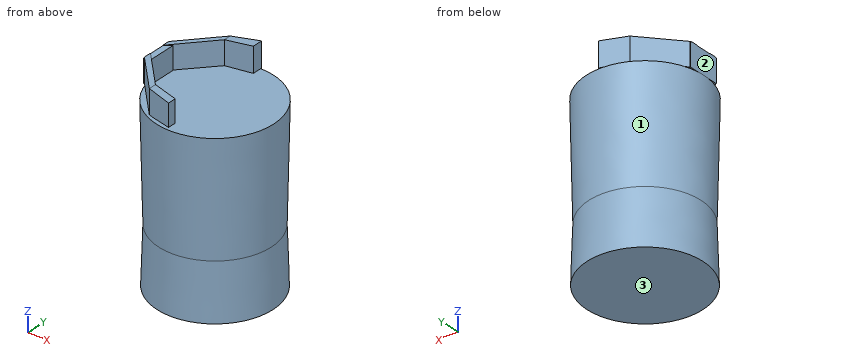
```python
from build123d import *

# Parameters (mm, degrees)
F10_R      = 51.6766678949
F9_R       = 49.5177054899
F14_R      = 51.0900787087
F11_FACE_R = 49.5177054899
F17_W      = 28.0700735748
F17_H      = 20.5879807472
F20_W      = 25.325415656
F20_H      = 19.9093073606
F23_W      = 6.3016116619
F23_H      = 20.8089984953
F22_W      = 6.4192367718
F22_H      = 20.5292478204
F22_W_2    = 6.6290111281
F22_H_2    = 20.7466594875
F23_W_2    = 6.6997222602
F23_H_2    = 21.3462822139
F26_W      = 7.3063448071
F26_H      = 19.5261649787
F28_W      = 9.0555027127
F28_H      = 21.7844322324


with BuildPart() as f11:
    # F10 (on face) → F11 section 0
    with BuildSketch(Plane.XY.offset(50.2420156263)):
        Circle(F10_R)
    # F9 (on face) → F11 section 1
    with BuildSketch(Plane.XY.offset(-49.2490320466)):
        Circle(F9_R)
    loft()

    # F14 (on offset) → F15 section 0
    with BuildSketch(Plane.XY.offset(-98.71355223)):
        Circle(F14_R)
    # F11_face (on face) → F15 section 1
    with BuildSketch(Plane(origin=(0, 0, -49.2490320466), x_dir=(1, 0, 0), z_dir=(0, 0, -1))):
        Circle(F11_FACE_R)
    loft()

    # F17 (on offset) → F21 section 0
    with BuildSketch(Plane.YZ.offset(-51.4408089221)):
        with Locations((-0.1785028726, 60.4957193136)):
            Rectangle(F17_W, F17_H)
    # F20 (on offset) → F21 section 1
    with BuildSketch(Plane.YZ.offset(-46.7405449599)):
        with Locations((-0.1616971567, 60.256190598)):
            Rectangle(F20_W, F20_H)
    loft()

    # F23 (on offset) → F24 section 0
    with BuildSketch(Plane.YZ.offset(-22.4701166153)):
        with Locations((41.3124375045, 61.3829698414)):
            Rectangle(F23_W, F23_H)
    # F22 (on offset) → F24 section 1
    with BuildSketch(Plane.YZ.offset(-51.4408089221)):
        with Locations((9.9052698351, 60.8711652458)):
            Rectangle(F22_W, F22_H)
    loft()

    # F22 (on offset) → F25 section 0
    with BuildSketch(Plane.YZ.offset(-51.4408089221)):
        with Locations((-10.0758362096, 60.7760790735)):
            Rectangle(F22_W_2, F22_H_2)
    # F23 (on offset) → F25 section 1
    with BuildSketch(Plane.YZ.offset(-22.4701166153)):
        with Locations((-40.5898671597, 60.6302414089)):
            Rectangle(F23_W_2, F23_H_2)
    loft()

    # F23 (on offset) → F27 section 0
    with BuildSketch(Plane.YZ.offset(-22.4701166153)):
        with Locations((-40.5898671597, 60.6302414089)):
            Rectangle(F23_W_2, F23_H_2)
    # F26 (on Right) → F27 section 1
    with BuildSketch(Plane.YZ):
        with Locations((-47.1889227629, 61.6251770407)):
            Rectangle(F26_W, F26_H)
    loft()

    # F28 (on Right) → F29 section 0
    with BuildSketch(Plane.YZ):
        with Locations((46.41026631, 62.4425597489)):
            Rectangle(F28_W, F28_H)
    # F23 (on offset) → F29 section 1
    with BuildSketch(Plane.YZ.offset(-22.4701166153)):
        with Locations((41.3124375045, 61.3829698414)):
            Rectangle(F23_W, F23_H)
    loft()


solid = f11.part
```
Geometry check sheet. Reference: the model listing, model coordinates, mm. Face numbers are marked on the shaded views. Round coordinates to 2 decimals unless told otherwise and drop trailing zeros. Order: outer loops, then holes, each group sorted by start corner. A loop starts at its lowest first (then second) coordinate and runs counter-clockwise, first axis right, second up. Notation, with made-up numbers: (-13.75, -17) -> (33.25, -17) arc R10 cw to (33.25, -7) -> close; hole circle Ø2 at (-13, 81). An arc over 180 degrees is marked (long way). Return JSON: item names as keys, results as strings. Group by question number.
Q1. Section check B-B, the plane z = 15. Record the boundary of the cut face in (x, y), plus the area to 3 significant figures.
Q2. Gauge pin test, flat ends, axial feed: pin 1 (1.5 mm diameter, centred on x = -22.5, z = 12, fed in from +Y); pin 2 (3.5 mm diameter, centred on y = -49, z = 61, fed in from +X); pin 3 (12 mm diameter, centred on x = 36.5, z = 11.5, fed in from +Y). Record the tip position at first contact, or that the pin passes through.
Q3. Section check A-A, the plane z = -35. Record the boundary of the cut face in (x, y), plus the area to 3 significant figures.
Q4. Release check for a two-part mould opening along Z. For the marked faces 1, 2 and 3 record: released by +Z, released by -Z, zero draft, split by the parting line, or undercut.
Q5. Material ranges on probe 1 along Z at (x, y) = (24, -23); probe 2 along X at (y, z) = (3.5, 54); probe 3 along X at (y, z) = (4.5, -42.5), recorded low to high. Write a range as from..to.
Numbers:
{
 "1": {"outline": "circle Ø101.82 at (0, 0)", "area": "8,140 mm^2"},
 "2": {"pin 1": "y = 45.96", "pin 2": "x = 0", "pin 3": "y = 40.67"},
 "3": {"outline": "circle Ø99.65 at (0, 0)", "area": "7,800 mm^2"},
 "4": {"face 1": "undercut", "face 2": "zero draft", "face 3": "released by -Z"},
 "5": {"probe 1": "-98.71..50.24", "probe 2": "-51.44..-46.74", "probe 3": "-49.46..49.46"}
}
